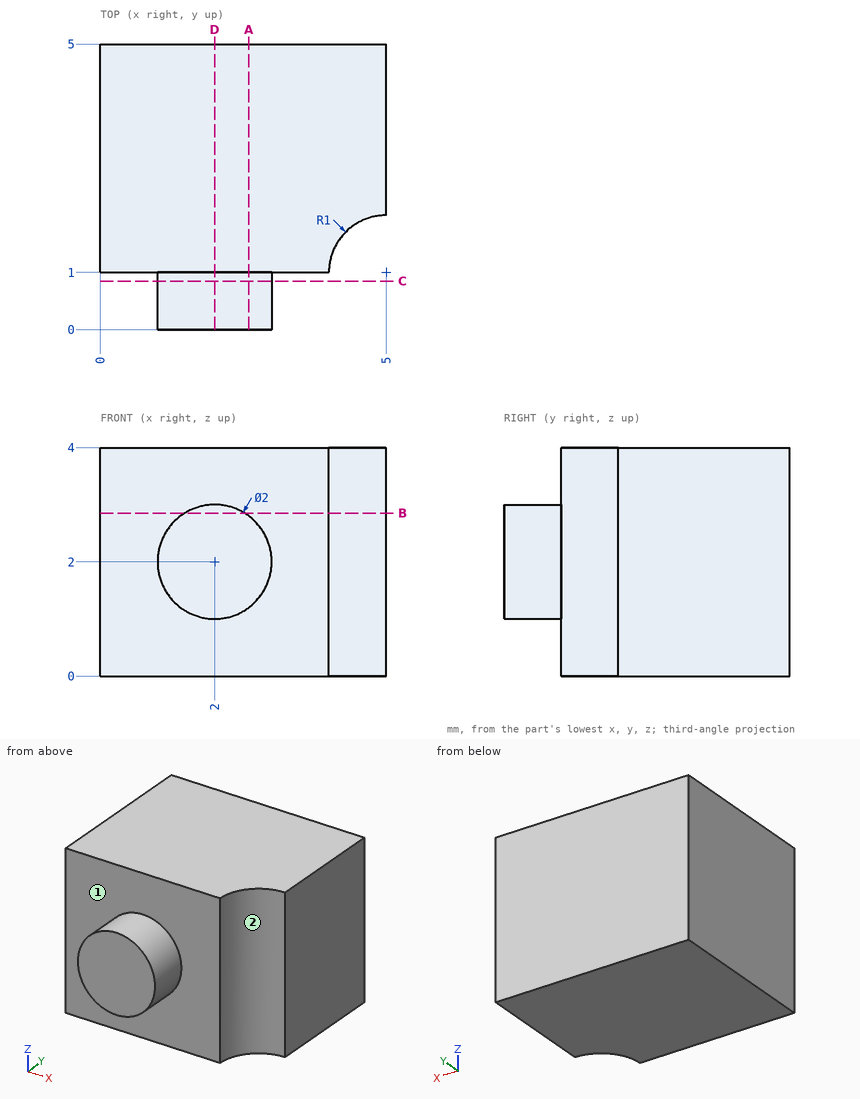
Drawing for the job (mm, zero at the part's lowest x, y, z). A direction names the side the tool comes from. Round coordinates to 2 decimals unless told otherwise and drop trailing zeros. Loops run counter-clockwise (first coordinate to the right, second up) from the corner with the lowest first, then second, coordinate; pieces in that order, holes last. Notation, with made-up numbers: (46, 85) - (53, 85) arc R17 cw to (53, 102) - close; hole circle Ø8 at (61.25, 73.5). An arc over 180 degrees is marked (long way). Write each question's results on one line, items separated by ' | '.
(1) Wall check: L1, parallel to Y at x = 0.7, z = 1.65; L2, parallel to Z at x = 2, y = 0.95; L3, parallel to X at y = 1.1, z = 1.05. Give the ranges that are in metal, low to high.
Answer below:
L1: y = 1 to 5 | L2: z = 1 to 3 | L3: x = 0 to 4.01
(2) Saw through at A-A, the plane x = 2.6. List the corners of the cut face in (y, z), then the cut area to 3 significant figures.
Answer below:
outline: (0, 1.2) - (1, 1.2) - (1, 0) - (5, 0) - (5, 4) - (1, 4) - (1, 2.8) - (0, 2.8) - close | area: 17.6 mm^2
(3) Saw through at B-B, the plane z = 2.85. List the corners of the cut face in (x, y).
Answer below:
outline: (0, 1) - (1.47, 1) - (1.47, 0) - (2.53, 0) - (2.53, 1) - (4, 1) arc R1 cw to (5, 2) - (5, 5) - (0, 5) - close
(4) 3-axis set-ups, long thin cutter, end or side, ignore diameter. For the marked faces 1 and 2: which of +Z, -Z, +X, -X, +Y, -Y reach the whole face in a straight line?
Answer below:
face 1: -Y | face 2: +Z, -Z, +X, -Y
(5) Saw through at C-C, the plane y = 0.85. List the corners of the cut face in (x, z).
Answer below:
outline: circle Ø2 at (2, 2)
(6) Saw through at D-D, the plane x = 2. List the corners of the cut face in (y, z).
Answer below:
outline: (0, 1) - (1, 1) - (1, 0) - (5, 0) - (5, 4) - (1, 4) - (1, 3) - (0, 3) - close
